Check sheet for the drawn part. Datum: minimum x, y, z corner. Units: mm. A direction names the side the tool comes from. Coordinates: 2 decimals unless noted, no trailing zeros. Order: outer loops, then holes, each group sorted by start corner. A loop starts at its lowest first (then second) coordinate and runs counter-clockwise, first axis right, second up.
1. Draft check along X on the marked faces 4, 5, 6 and 7. Enter one of: released by +X, released by -X, zero draft, split by the parting line, or undercut.
2. Set-up check for the marked faces 1, 2 and 3: record each of +Z, -Z, +X, -X, +Y, -Y from which the full face is reachable in a straight line by a thin tool's end or side.
3. Cross-section at D-D (x = 31.5). Enter the section's corners in (y, z), then the cut area to 4 significant figures.
4. Cross-section at B-B (y = 6.75). Enter the section's corners in (x, z).
5. Thickness scan on line 1 (Y direction, x = 47.5, z = 4.5); line 2 (Y direction, x = 51.5, z = 3); line 3 (Z direction, x = 18.5, y = 2.5). Record the ranges inside material, lowest first.
6. Cross-section at A-A (z = 5.25). Enter the section's corners in (x, y).
7. Cross-section at C-C (z = 10.75). Count the separate pieces of the cut face and the enclosed holes in it.
8. Gauge pin test, flat ends, axial feed: pin 1 Ø1.5 at (x, y) = (43.5, 13.5) entering from -Z; pin 2 Ø1.6 at (x, y) = (7.5, 7.5) entering from +Z; pin 3 Ø2 at (x, z) = (12.5, 1.5) entering from -Y; pin 4 Ø5.5 at (x, y) = (20, 6) entering from -Z. Record the tip position at first contact, or that the pin passes through.
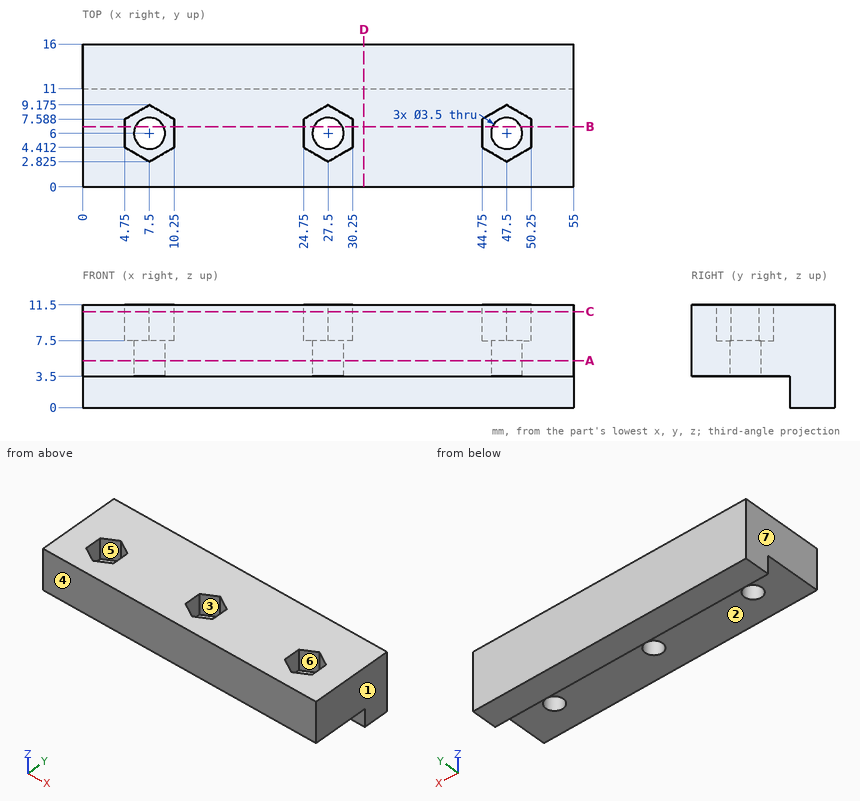
Data:
1. face 4: zero draft
1. face 5: undercut
1. face 6: undercut
1. face 7: released by -X
2. face 1: +Z, -Z, +X, +Y, -Y
2. face 2: -Z, +X, -X, -Y
2. face 3: +Z
3. outline: (0, 3.5) - (11, 3.5) - (11, 0) - (16, 0) - (16, 11.5) - (0, 11.5) - close
3. area: 145.5 mm2
4. outline: (0, 3.5) - (5.92, 3.5) - (5.92, 7.5) - (4.75, 7.5) - (4.75, 11.5) - (0, 11.5) - close; (9.08, 3.5) - (25.92, 3.5) - (25.92, 7.5) - (24.75, 7.5) - (24.75, 11.5) - (10.25, 11.5) - (10.25, 7.5) - (9.08, 7.5) - close; (29.08, 3.5) - (45.92, 3.5) - (45.92, 7.5) - (44.75, 7.5) - (44.75, 11.5) - (30.25, 11.5) - (30.25, 7.5) - (29.08, 7.5) - close; (49.08, 3.5) - (55, 3.5) - (55, 11.5) - (50.25, 11.5) - (50.25, 7.5) - (49.08, 7.5) - close
5. line 1: y = 0 to 4.25, 7.75 to 16
5. line 2: y = 11 to 16
5. line 3: z = 3.5 to 11.5
6. outline: (0, 0) - (55, 0) - (55, 16) - (0, 16) - close; hole circle Ø3.5 at (7.5, 6); hole circle Ø3.5 at (27.5, 6); hole circle Ø3.5 at (47.5, 6)
7. separate pieces: 1
7. enclosed holes: 3
8. pin 1: stops at z = 0
8. pin 2: stops at z = 7.5
8. pin 3: stops at y = 11
8. pin 4: stops at z = 3.5
